Autodesk Inventor part; units mm, degrees
ref_plane "YZ Plane" through (0, 0, 0) normal (1, 0, 0) x (0, 1, 0)
ref_plane "XZ Plane" through (0, 0, 0) normal (0, 1, 0) x (-1, 0, 0)
ref_plane "XY Plane" through (0, 0, 0) normal (0, 0, 1) x (1, 0, 0)
sketch "Sketch1" plane through (0, 0, 0) normal (0, 0, 1) x (1, 0, 0)
  line L0 (2.794, -4.191) -> (2.794, -3.429)
  line L1 (2.794, -3.429) -> (3.556, -3.429)
  line L2 (3.556, -3.429) -> (3.556, -4.191)
  line L3 (3.556, -4.191) -> (2.794, -4.191)
  line L4 (2.794, -6.731) -> (2.794, -5.969)
  line L5 (2.794, -5.969) -> (3.556, -5.969)
  line L6 (3.556, -5.969) -> (3.556, -6.731)
  line L7 (3.556, -6.731) -> (2.794, -6.731)
  line L8 (2.794, -1.651) -> (2.794, -0.889)
  line L9 (2.794, -0.889) -> (3.556, -0.889)
  line L10 (3.556, -0.889) -> (3.556, -1.651)
  line L11 (3.556, -1.651) -> (2.794, -1.651)
  line L12 (5.334, 0) -> (5.334, -7.62)
  line L13 (5.334, 0) -> (0, 0)
  line L14 (0, 0) -> (0, -7.62)
  line L15 (0, -7.62) -> (5.334, -7.62)
  line L16 (5.334, -7.62) -> (6.35, -7.62)
  line L17 (6.35, 0) -> (6.35, -7.62)
  line L18 (6.35, 0) -> (5.334, 0)
  line L19 (-0.611, -8.231) -> (-0.611, 0.611)
  line L20 (-0.611, 0.611) -> (5.334, 0.611)
  line L21 (5.334, 0.611) -> (6.961, 0.611)
  line L22 (6.961, 0.611) -> (6.961, -8.231)
  line L23 (6.961, -8.231) -> (5.334, -8.231)
  line L24 (5.334, -8.231) -> (-0.611, -8.231)
  point P0 (-0.635, 26.67)
  dimension "d2" = 0.611
extrude "Extrusion1" add sketch "Sketch1" along normal blind 5.0038 contours L18 L17 L16 L12 | L12 L15 L14 L13
sketch "Sketch2" plane through (0, -7.62, 0) normal (0, -1, 0) x (1, 0, 0)
  point P0 (-0.635, -6.0808)
sketch "Sketch3" plane through (0, -7.62, 0) normal (0, -1, 0) x (1, 0, 0)
  line L0 (6.35, 5.0038) -> (6.35, 0)
  line L1 (5.334, 5.0038) -> (6.35, 5.0038)
  line L2 (4.6228, 3.3857) -> (5.334, 5.0038)
  line L3 (5.334, 1.7675) -> (4.6228, 3.3857)
  line L4 (5.334, 0) -> (5.334, 1.7675)
  line L5 (0, 0) -> (5.334, 0)
  line L6 (5.334, 0) -> (6.35, 0)
  point P0 (-0.635, -6.0808)
extrude "Extrusion2" cut sketch "Sketch3" against normal blind 25.4
ref_plane "Work Plane5" through (0, 0, 8.1788) normal (0, 0, 1) x (1, 0, 0)
ref_plane "Work Plane7" through (0, 0, 11.3538) normal (0, 0, 1) x (1, 0, 0)
ref_plane "Work Plane9" through (0, 0, 8.1788) normal (0, 0, 1) x (1, 0, 0)
ref_plane "Work Plane10" through (0, 0, 11.3538) normal (0, 0, 1) x (1, 0, 0)
ref_plane "Work Plane11" through (0, 0, 8.1788) normal (0, 0, 1) x (1, 0, 0)
ref_plane "Work Plane12" through (0, 0, 11.3538) normal (0, 0, 1) x (1, 0, 0)
sketch "Sketch4" plane through (0, 0, 5.0038) normal (0, 0, 1) x (1, 0, 0)
  line L0 (5.334, -7.62) -> (5.334, 0)
  line L1 (0, 0) -> (5.334, 0)
  line L2 (0, -7.62) -> (0, 0)
  line L3 (5.334, -7.62) -> (0, -7.62)
  line L4 (2.794, -3.429) -> (3.556, -3.429)
  line L5 (3.556, -3.429) -> (3.556, -4.191)
  line L6 (3.556, -4.191) -> (2.794, -4.191)
  line L7 (2.794, -4.191) -> (2.794, -3.429)
  line L8 (2.794, -5.969) -> (3.556, -5.969)
  line L9 (3.556, -5.969) -> (3.556, -6.731)
  line L10 (3.556, -6.731) -> (2.794, -6.731)
  line L11 (2.794, -6.731) -> (2.794, -5.969)
  line L12 (2.794, -0.889) -> (3.556, -0.889)
  line L13 (3.556, -0.889) -> (3.556, -1.651)
  line L14 (3.556, -1.651) -> (2.794, -1.651)
  line L15 (2.794, -1.651) -> (2.794, -0.889)
extrude "Extrusion3" add sketch "Sketch4" along normal blind 6.35
ref_plane "Work Plane6" through (0, 0, 8.1788) normal (0, 0, 1) x (1, 0, 0)
ref_plane "Work Plane8" through (0, 0, 11.3538) normal (0, 0, 1) x (1, 0, 0)
properties part number "pwm connector"
Read the model definition and answer for the solid it produces. Units are mm, in the model's axes. A direction names the side the tool comes from. Round coordinates to 2 decimals unless told otherwise and drop trailing zeros. Loops run counter-clockwise (first coordinate to the right, second up) from the corner with the lowest first, then second, coordinate; pieces in that order, holes last.
Q1. Section C-C on z = 9.25 is taken. Write down the section's boundary in (x, y), and give its area (3 significant figures).
Q2. Which of the six approach directions +Z, -Z, +X, -X, +Y, -Y give full straight-line access (tool end or side, diameter ignored) to faces 1 (the face through (3, -7.62, 6)), 2 (the face through (4.98, -3.86, 2.57))?
Q3. Section A-A on x = 3.4 is taken. Write down the section's boundary in (y, z), and give its area (3 significant figures).
Q4. Section D-D on y = -0.75 is taken. Write down the section's boundary in (x, z).
Q5. Consider probe 1 along Y at (x, z) = (3.2, 5); probe 2 along X at (y, z) = (-1.5, 10.75); probe 3 along Z at (x, y) = (5.05, -4). Determine where each line is inside the solid, lowest interval first.
Q6. Section B-B on y = -4 is taken. Write down the section's boundary in (x, z), and give its area (3 significant figures).
Q7. This flat-tipped pin is pushed along its axis until it touches: pin 1 (0.8 mm diameter, centred on x = 3, z = 7, fed in from +Y). Where does it stop, or does it pass through?
Output:
1. outline: (0, -7.62) - (5.33, -7.62) - (5.33, 0) - (0, 0) - close; hole (2.79, -6.73) - (3.56, -6.73) - (3.56, -5.97) - (2.79, -5.97) - close; hole (2.79, -4.19) - (3.56, -4.19) - (3.56, -3.43) - (2.79, -3.43) - close; hole (2.79, -1.65) - (3.56, -1.65) - (3.56, -0.89) - (2.79, -0.89) - close
1. area: 38.9 mm2
2. face 1: +Z, -Z, +X, -X, -Y
2. face 2: +X, +Y, -Y
3. outline: (-7.62, 0) - (-6.73, 0) - (-6.73, 11.35) - (-7.62, 11.35) - close; (-5.97, 0) - (-4.19, 0) - (-4.19, 11.35) - (-5.97, 11.35) - close; (-3.43, 0) - (-1.65, 0) - (-1.65, 11.35) - (-3.43, 11.35) - close; (-0.89, 0) - (0, 0) - (0, 11.35) - (-0.89, 11.35) - close
3. area: 60.6 mm2
4. outline: (0, 0) - (5.33, 0) - (5.33, 1.77) - (4.62, 3.39) - (5.33, 5) - (5.33, 11.35) - (0, 11.35) - close
5. probe 1: y = -7.62 to -6.73, -5.97 to -4.19, -3.43 to -1.65, -0.89 to 0
5. probe 2: x = 0 to 2.79, 3.56 to 5.33
5. probe 3: z = 0 to 2.41, 4.36 to 11.35
6. outline: (0, 0) - (2.79, 0) - (2.79, 11.35) - (0, 11.35) - close; (3.56, 0) - (5.33, 0) - (5.33, 1.77) - (4.62, 3.39) - (5.33, 5) - (5.33, 11.35) - (3.56, 11.35) - close
6. area: 50.8 mm2
7. pin 1: stops at y = 0
